from build123d import *

# Parameters (mm, degrees)
F0_W     = 50
F0_H     = 15
F1_DEPTH = 60
F2_T     = -1
F3_R     = 1.5


with BuildPart() as f1:
    # F0 (on Top) → F1 (new body)
    with BuildSketch(Plane.XY):
        Rectangle(F0_W, F0_H)
    extrude(amount=F1_DEPTH)

    # F2
    f2_openings = [f1.faces().sort_by_distance(p)[0] for p in [
        (0, 0, 60),
        (0, 0, 0),
    ]]
    offset(amount=F2_T, openings=f2_openings)

    # F3
    f3_edges = [f1.edges().sort_by_distance(p)[0] for p in [
        (25, 7.5, 30),
        (25, -7.5, 30),
        (-25, 7.5, 30),
        (-25, -7.5, 30),
        (-24, -6.5, 30),
        (24, -6.5, 30),
        (-24, 6.5, 30),
        (24, 6.5, 30),
    ]]
    fillet(f3_edges, radius=F3_R)


solid = f1.part
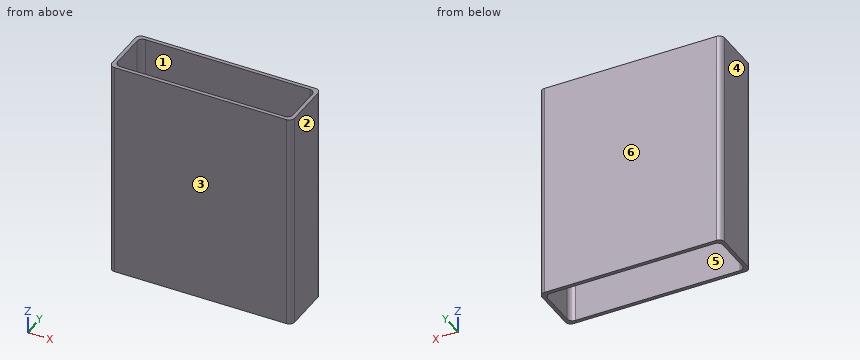
Geometry check sheet. Reference: the model listing, model coordinates, mm. Face numbers are marked on the shaded views. A direction names the side the tool comes from. Give positions to 0.01 mm unless a question says otherwise; leave off trailing zeros. Loops run counter-clockwise (first coordinate to the right, second up) from the corner with the lowest first, then second, coordinate; pieces in that order, holes last. Notation, with made-up numbers: (29.25, -33.5) -> (39.25, -33.5) arc R16 cw to (39.25, -21.5) -> close; hole circle Ø1 at (32, -24). An arc over 180 degrees is marked (long way). Answer in a Markdown table with one row per item. Add a question column.
1) Draft check along Y on the marked faces 3, 4, 5 and 6. Enter one of: pulls with the +Y half, pulls with the -Y half, needs draft (parallel to the pull), parting line crosses it, or undercut.
2) Cross-section at B-B on x = -16. Record the boundary of the cut face in (y, z), and give its area (3 significant figures).
3) Set-up check for the marked faces 1 and 2: record each of +Z, -Z, +X, -X, +Y, -Y from which the full face is reachable in a straight line by a thin tool's end or side.
4) Cross-section at A-A on y = 4. Record the boundary of the cut face in (x, z).
5) Cross-section at C-C on z = 19.5. Record the boundary of the cut face in (x, y), and give its area (3 significant figures).
6) Material ranges on probe 1 along Y at (x, z) = (2, 10); probe 2 along X at (y, z) = (-2.75, 31); probe 3 along Y at (x, z) = (-23, 47), recorded low to high. Write a range as from..to.
Outcome:
| question | item | result |
|---|---|---|
| 1 | face 3 | pulls with the -Y half |
| 1 | face 4 | needs draft |
| 1 | face 5 | undercut |
| 1 | face 6 | pulls with the +Y half |
| 2 | outline | (-7.5, 0) -> (-6.5, 0) -> (-6.5, 60) -> (-7.5, 60) -> close; (6.5, 0) -> (7.5, 0) -> (7.5, 60) -> (6.5, 60) -> close |
| 2 | area | 120 mm^2 |
| 3 | face 1 | +Z, -Z |
| 3 | face 2 | +Z, -Z, +X, +Y, -Y |
| 4 | outline | (-25, 0) -> (-24, 0) -> (-24, 60) -> (-25, 60) -> close; (24, 0) -> (25, 0) -> (25, 60) -> (24, 60) -> close |
| 5 | outline | (-25, -6) arc R1.5 ccw to (-23.5, -7.5) -> (23.5, -7.5) arc R1.5 ccw to (25, -6) -> (25, 6) arc R1.5 ccw to (23.5, 7.5) -> (-23.5, 7.5) arc R1.5 ccw to (-25, 6) -> close; hole (-24, -5) arc R1.5 ccw to (-22.5, -6.5) -> (22.5, -6.5) arc R1.5 ccw to (24, -5) -> (24, 5) arc R1.5 ccw to (22.5, 6.5) -> (-22.5, 6.5) arc R1.5 ccw to (-24, 5) -> close |
| 5 | area | 126 mm^2 |
| 6 | probe 1 | y = -7.5..-6.5, 6.5..7.5 |
| 6 | probe 2 | x = -25..-24, 24..25 |
| 6 | probe 3 | y = -7.5..-6.41, 6.41..7.5 |
